from build123d import *


with BuildPart() as f1:
    # F0 (on Right) → F1 (revolve)
    with BuildSketch(Plane.YZ):
        with BuildLine():
            Line((0, -89.237345), (0, -10.442538))
            ThreePointArc((0, -10.442538), (-25.539414, -7.80404), (-50, 0))
            Line((-50, 0), (-98.031412, 45.791994))
            ThreePointArc((-98.031412, 45.791994), (-108, 55), (-117.968588, 45.791994))
            Line((-117.968588, 45.791994), (-121, 45.791994))
            Line((-121, 45.791994), (-121, 50.762655))
            Line((-121, 50.762655), (-133, 50.762655))
            Line((-133, 50.762655), (-133, 38.762655))
            Line((-133, 38.762655), (-115.75, 38.762655))
            Line((-115.75, 38.762655), (-115.75, 28.762655))
            Line((-115.75, 28.762655), (-107.782677, 28.762655))
            Line((-107.782677, 28.762655), (-82.250395, -35.764394))
            Line((-82.250395, -35.764394), (-72.037482, -35.764394))
            Line((-72.037482, -35.764394), (-72.037482, -41.503783))
            Line((-72.037482, -41.503783), (-90.14219, -41.503783))
            Line((-90.14219, -41.503783), (-90.14219, -82.738219))
            Line((-90.14219, -82.738219), (-81.00698, -82.738219))
            Line((-81.00698, -82.738219), (-81.00698, -89.237345))
            Line((-81.00698, -89.237345), (0, -89.237345))
        make_face()
    revolve(axis=Axis((0, 0, -49.839942), (0, 0, -1)))


solid = f1.part
Can you work these out from the model? Positions are in its coordinate system, mm. A direction names the side the tool comes from. Coordinates: 2 decimals unless noted, no trailing zeros. Order: outer loops, then holes, each group sorted by start corner. A loop starts at its lowest first (then second) coordinate and runs counter-clockwise, first axis right, second up. Notation, with made-up numbers: M 55,-1.5 L 65,-1.5 A12 cw 65,2.5 Z; hole C -27,34.5 d7. An arc over 180 degrees is marked long. Answer as CSV lines item,"result".
(1) If we mould it in two halves opening along Z, with no side actions, what happens to faces 1 (the flat face through (40, -61, -41.504)), 2 (the flat face through (116, 26, 45.792)), 3 (the flat face through (-34, 74, -82.738))? For each: released by +Z, released by -Z, zero draft, split by the parting line, or undercut.
Geometry check:
face 1,"undercut"
face 2,"released by +Z"
face 3,"released by -Z"
(2) On a 3-axis mill with a long thin cutter (end or side, diameter ignored), from which of +Z, -Z, +X, -X, +Y, -Y can I reach the whole of each face in a straight line? I mean faces 4 (the flat face through (118, 29, 50.763)), 5 (the flat face through (-109, 40, 38.763)), 6 (the cylindrical face through (43.83, 57.17, -38.67)). Say none if no direction works.
Geometry check:
face 4,"+Z"
face 5,"-Z"
face 6,"none"
(3) Please list where these lines run through material, in increasing order: L1, parallel to Y at x = 0, z = 49; L2, parallel to X at y = 0, z = 49.75; L3, parallel to Y at x = 0, z = 47.35.
Geometry check:
L1,"-133 to -121, -117.17 to -98.83, 98.83 to 117.17, 121 to 133"
L2,"-133 to -121, -116.8 to -99.2, 99.2 to 116.8, 121 to 133"
L3,"-133 to -121, -117.72 to -98.28, 98.28 to 117.72, 121 to 133"
(4) I'm going to push flat-ended pins straight in: pin 1 (6 mm diameter, centred on x = 68, y = 104, fed in from +Z); pin 2 (4 mm diameter, centred on x = 77, z = -13.5, fed in from -Y); pin 3 (1.5 mm diameter, centred on x = -10.5, z = 20.5, fed in from -Y); pin 4 (4 mm diameter, centred on y = -93, z = -72, fed in from +X). Where does each tip first touch, or does it pass through?
Geometry check:
pin 1,"z = 50.76"
pin 2,"y = -51.96"
pin 3,"y = -104.29"
pin 4,"through"
(5) Suppose I cut it at A-A on z = -74. Please give me the cut outline in (x, y), plus the area to 3 significant figures.
Geometry check:
outline,"C 0,0 d180.28"
area,"25,500 mm^2"
